from build123d import *
from OCP.BRepFilletAPI import BRepFilletAPI_MakeChamfer

# Parameters (mm, degrees)
BOSS_EXTRUDE1_DEPTH         = 2.29
SKETCH3_W                   = 0.64
SKETCH3_H                   = 0.64
CHAMFER3_SIZE               = 0.5
CHAMFER3_SIZE2              = 0.133974596
LPATTERN1_COUNT             = 5
LPATTERN1_PITCH             = 2.54
CHAMFER3_OF_LPATTERN1_SIZE  = 0.5
CHAMFER3_OF_LPATTERN1_SIZE2 = 0.133974596


with BuildPart() as part:
    # Sketch1 → Boss-Extrude1 (new body)
    with BuildSketch(Plane(origin=(0, 0, 0), x_dir=(1, 0, 0), z_dir=(0, 1, 0))):
        Polygon((-0.77, 1.25), (0.77, 1.25), (1.25, 0.75), (1.27, 0.75), (1.27, -0.75), (1.25, -0.75), (0.77, -1.25), (-0.77, -1.25), (-1.25, -0.75), (-1.27, -0.75), (-1.27, 0.75), (-1.25, 0.75), align=None)
    boss_extrude1 = extrude(amount=BOSS_EXTRUDE1_DEPTH)

    # Sweep1: sweep along a path in Sketch2
    with BuildLine(Plane(origin=(0, 0, 0), x_dir=(0, 0, -1), z_dir=(1, 0, 0))) as sweep1_path:
        Line((0, 8.13), (0, -0.408142235))
        ThreePointArc((0, -0.408142235), (-0.095150584, -0.886496526), (-0.366116524, -1.292025712))
        Line((-0.366116524, -1.292025712), (-2.124090812, -3.05))
    # Sketch3 → Sweep1 (sweep)
    with BuildSketch(Plane(origin=(0, 8.13, 0), x_dir=(1, 0, 0), z_dir=(0, 1, 0))):
        Rectangle(SKETCH3_W, SKETCH3_H)
    sweep1 = sweep(path=sweep1_path.line)

    # Chamfer3: one chamfer whose edges measure the first distance from different faces: ONE call of the kernel's chamfer builder (chamfer() names one face for all edges)
    chamfer3_edges_1 = [part.edges().sort_by_distance(p)[0] for p in [
        (0.32, 8.13, 0),
    ]]
    chamfer3_side_1 = [part.faces().sort_by_distance(p)[0] for p in [
        (0.32, 5.21, 0),
    ]]
    chamfer3_edges_2 = [part.edges().sort_by_distance(p)[0] for p in [
        (0, 8.13, -0.32),
    ]]
    chamfer3_side_2 = [part.faces().sort_by_distance(p)[0] for p in [
        (0, 5.21, -0.32),
    ]]
    chamfer3_edges_3 = [part.edges().sort_by_distance(p)[0] for p in [
        (-0.32, 8.13, 0),
    ]]
    chamfer3_side_3 = [part.faces().sort_by_distance(p)[0] for p in [
        (-0.32, 5.21, 0),
    ]]
    chamfer3_edges_4 = [part.edges().sort_by_distance(p)[0] for p in [
        (0, 8.13, 0.32),
    ]]
    chamfer3_side_4 = [part.faces().sort_by_distance(p)[0] for p in [
        (0, 5.21, 0.32),
    ]]
    chamfer3 = BRepFilletAPI_MakeChamfer(part.part.solid().wrapped)
    for e in chamfer3_edges_1:
        chamfer3.Add(CHAMFER3_SIZE, CHAMFER3_SIZE2, e.wrapped, chamfer3_side_1[0].wrapped)  # the first distance lies on this face
    for e in chamfer3_edges_2:
        chamfer3.Add(CHAMFER3_SIZE, CHAMFER3_SIZE2, e.wrapped, chamfer3_side_2[0].wrapped)  # the first distance lies on this face
    for e in chamfer3_edges_3:
        chamfer3.Add(CHAMFER3_SIZE, CHAMFER3_SIZE2, e.wrapped, chamfer3_side_3[0].wrapped)  # the first distance lies on this face
    for e in chamfer3_edges_4:
        chamfer3.Add(CHAMFER3_SIZE, CHAMFER3_SIZE2, e.wrapped, chamfer3_side_4[0].wrapped)  # the first distance lies on this face
    add(Compound.cast(chamfer3.Shape()), mode=Mode.REPLACE)

    # LPattern1: Boss-Extrude1, Sweep1 ×5
    with Locations(*[(i * LPATTERN1_PITCH, 0, 0) for i in range(1, LPATTERN1_COUNT)]):
        add(boss_extrude1)
        add(sweep1)

    # Chamfer3 of LPattern1: one chamfer whose edges measure the first distance from different faces: ONE call of the kernel's chamfer builder (chamfer() names one face for all edges)
    chamfer3_of_lpattern1_edges_1 = [part.edges().sort_by_distance(p)[0] for p in [
        (2.86, 8.13, 0),
    ]]
    chamfer3_of_lpattern1_side_1 = [part.faces().sort_by_distance(p)[0] for p in [
        (2.86, 5.21, 0),
    ]]
    chamfer3_of_lpattern1_edges_2 = [part.edges().sort_by_distance(p)[0] for p in [
        (2.54, 8.13, -0.32),
    ]]
    chamfer3_of_lpattern1_side_2 = [part.faces().sort_by_distance(p)[0] for p in [
        (2.54, 5.21, -0.32),
    ]]
    chamfer3_of_lpattern1_edges_3 = [part.edges().sort_by_distance(p)[0] for p in [
        (2.22, 8.13, 0),
    ]]
    chamfer3_of_lpattern1_side_3 = [part.faces().sort_by_distance(p)[0] for p in [
        (2.22, 5.21, 0),
    ]]
    chamfer3_of_lpattern1_edges_4 = [part.edges().sort_by_distance(p)[0] for p in [
        (2.54, 8.13, 0.32),
    ]]
    chamfer3_of_lpattern1_side_4 = [part.faces().sort_by_distance(p)[0] for p in [
        (2.54, 5.21, 0.32),
    ]]
    chamfer3_of_lpattern1_edges_5 = [part.edges().sort_by_distance(p)[0] for p in [
        (5.4, 8.13, 0),
    ]]
    chamfer3_of_lpattern1_side_5 = [part.faces().sort_by_distance(p)[0] for p in [
        (5.4, 5.21, 0),
    ]]
    chamfer3_of_lpattern1_edges_6 = [part.edges().sort_by_distance(p)[0] for p in [
        (5.08, 8.13, -0.32),
    ]]
    chamfer3_of_lpattern1_side_6 = [part.faces().sort_by_distance(p)[0] for p in [
        (5.08, 5.21, -0.32),
    ]]
    chamfer3_of_lpattern1_edges_7 = [part.edges().sort_by_distance(p)[0] for p in [
        (4.76, 8.13, 0),
    ]]
    chamfer3_of_lpattern1_side_7 = [part.faces().sort_by_distance(p)[0] for p in [
        (4.76, 5.21, 0),
    ]]
    chamfer3_of_lpattern1_edges_8 = [part.edges().sort_by_distance(p)[0] for p in [
        (5.08, 8.13, 0.32),
    ]]
    chamfer3_of_lpattern1_side_8 = [part.faces().sort_by_distance(p)[0] for p in [
        (5.08, 5.21, 0.32),
    ]]
    chamfer3_of_lpattern1_edges_9 = [part.edges().sort_by_distance(p)[0] for p in [
        (7.94, 8.13, 0),
    ]]
    chamfer3_of_lpattern1_side_9 = [part.faces().sort_by_distance(p)[0] for p in [
        (7.94, 5.21, 0),
    ]]
    chamfer3_of_lpattern1_edges_10 = [part.edges().sort_by_distance(p)[0] for p in [
        (7.62, 8.13, -0.32),
    ]]
    chamfer3_of_lpattern1_side_10 = [part.faces().sort_by_distance(p)[0] for p in [
        (7.62, 5.21, -0.32),
    ]]
    chamfer3_of_lpattern1_edges_11 = [part.edges().sort_by_distance(p)[0] for p in [
        (7.3, 8.13, 0),
    ]]
    chamfer3_of_lpattern1_side_11 = [part.faces().sort_by_distance(p)[0] for p in [
        (7.3, 5.21, 0),
    ]]
    chamfer3_of_lpattern1_edges_12 = [part.edges().sort_by_distance(p)[0] for p in [
        (7.62, 8.13, 0.32),
    ]]
    chamfer3_of_lpattern1_side_12 = [part.faces().sort_by_distance(p)[0] for p in [
        (7.62, 5.21, 0.32),
    ]]
    chamfer3_of_lpattern1_edges_13 = [part.edges().sort_by_distance(p)[0] for p in [
        (10.48, 8.13, 0),
    ]]
    chamfer3_of_lpattern1_side_13 = [part.faces().sort_by_distance(p)[0] for p in [
        (10.48, 5.21, 0),
    ]]
    chamfer3_of_lpattern1_edges_14 = [part.edges().sort_by_distance(p)[0] for p in [
        (10.16, 8.13, -0.32),
    ]]
    chamfer3_of_lpattern1_side_14 = [part.faces().sort_by_distance(p)[0] for p in [
        (10.16, 5.21, -0.32),
    ]]
    chamfer3_of_lpattern1_edges_15 = [part.edges().sort_by_distance(p)[0] for p in [
        (9.84, 8.13, 0),
    ]]
    chamfer3_of_lpattern1_side_15 = [part.faces().sort_by_distance(p)[0] for p in [
        (9.84, 5.21, 0),
    ]]
    chamfer3_of_lpattern1_edges_16 = [part.edges().sort_by_distance(p)[0] for p in [
        (10.16, 8.13, 0.32),
    ]]
    chamfer3_of_lpattern1_side_16 = [part.faces().sort_by_distance(p)[0] for p in [
        (10.16, 5.21, 0.32),
    ]]
    chamfer3_of_lpattern1 = BRepFilletAPI_MakeChamfer(part.part.solid().wrapped)
    for e in chamfer3_of_lpattern1_edges_1:
        chamfer3_of_lpattern1.Add(CHAMFER3_OF_LPATTERN1_SIZE, CHAMFER3_OF_LPATTERN1_SIZE2, e.wrapped, chamfer3_of_lpattern1_side_1[0].wrapped)  # the first distance lies on this face
    for e in chamfer3_of_lpattern1_edges_2:
        chamfer3_of_lpattern1.Add(CHAMFER3_OF_LPATTERN1_SIZE, CHAMFER3_OF_LPATTERN1_SIZE2, e.wrapped, chamfer3_of_lpattern1_side_2[0].wrapped)  # the first distance lies on this face
    for e in chamfer3_of_lpattern1_edges_3:
        chamfer3_of_lpattern1.Add(CHAMFER3_OF_LPATTERN1_SIZE, CHAMFER3_OF_LPATTERN1_SIZE2, e.wrapped, chamfer3_of_lpattern1_side_3[0].wrapped)  # the first distance lies on this face
    for e in chamfer3_of_lpattern1_edges_4:
        chamfer3_of_lpattern1.Add(CHAMFER3_OF_LPATTERN1_SIZE, CHAMFER3_OF_LPATTERN1_SIZE2, e.wrapped, chamfer3_of_lpattern1_side_4[0].wrapped)  # the first distance lies on this face
    for e in chamfer3_of_lpattern1_edges_5:
        chamfer3_of_lpattern1.Add(CHAMFER3_OF_LPATTERN1_SIZE, CHAMFER3_OF_LPATTERN1_SIZE2, e.wrapped, chamfer3_of_lpattern1_side_5[0].wrapped)  # the first distance lies on this face
    for e in chamfer3_of_lpattern1_edges_6:
        chamfer3_of_lpattern1.Add(CHAMFER3_OF_LPATTERN1_SIZE, CHAMFER3_OF_LPATTERN1_SIZE2, e.wrapped, chamfer3_of_lpattern1_side_6[0].wrapped)  # the first distance lies on this face
    for e in chamfer3_of_lpattern1_edges_7:
        chamfer3_of_lpattern1.Add(CHAMFER3_OF_LPATTERN1_SIZE, CHAMFER3_OF_LPATTERN1_SIZE2, e.wrapped, chamfer3_of_lpattern1_side_7[0].wrapped)  # the first distance lies on this face
    for e in chamfer3_of_lpattern1_edges_8:
        chamfer3_of_lpattern1.Add(CHAMFER3_OF_LPATTERN1_SIZE, CHAMFER3_OF_LPATTERN1_SIZE2, e.wrapped, chamfer3_of_lpattern1_side_8[0].wrapped)  # the first distance lies on this face
    for e in chamfer3_of_lpattern1_edges_9:
        chamfer3_of_lpattern1.Add(CHAMFER3_OF_LPATTERN1_SIZE, CHAMFER3_OF_LPATTERN1_SIZE2, e.wrapped, chamfer3_of_lpattern1_side_9[0].wrapped)  # the first distance lies on this face
    for e in chamfer3_of_lpattern1_edges_10:
        chamfer3_of_lpattern1.Add(CHAMFER3_OF_LPATTERN1_SIZE, CHAMFER3_OF_LPATTERN1_SIZE2, e.wrapped, chamfer3_of_lpattern1_side_10[0].wrapped)  # the first distance lies on this face
    for e in chamfer3_of_lpattern1_edges_11:
        chamfer3_of_lpattern1.Add(CHAMFER3_OF_LPATTERN1_SIZE, CHAMFER3_OF_LPATTERN1_SIZE2, e.wrapped, chamfer3_of_lpattern1_side_11[0].wrapped)  # the first distance lies on this face
    for e in chamfer3_of_lpattern1_edges_12:
        chamfer3_of_lpattern1.Add(CHAMFER3_OF_LPATTERN1_SIZE, CHAMFER3_OF_LPATTERN1_SIZE2, e.wrapped, chamfer3_of_lpattern1_side_12[0].wrapped)  # the first distance lies on this face
    for e in chamfer3_of_lpattern1_edges_13:
        chamfer3_of_lpattern1.Add(CHAMFER3_OF_LPATTERN1_SIZE, CHAMFER3_OF_LPATTERN1_SIZE2, e.wrapped, chamfer3_of_lpattern1_side_13[0].wrapped)  # the first distance lies on this face
    for e in chamfer3_of_lpattern1_edges_14:
        chamfer3_of_lpattern1.Add(CHAMFER3_OF_LPATTERN1_SIZE, CHAMFER3_OF_LPATTERN1_SIZE2, e.wrapped, chamfer3_of_lpattern1_side_14[0].wrapped)  # the first distance lies on this face
    for e in chamfer3_of_lpattern1_edges_15:
        chamfer3_of_lpattern1.Add(CHAMFER3_OF_LPATTERN1_SIZE, CHAMFER3_OF_LPATTERN1_SIZE2, e.wrapped, chamfer3_of_lpattern1_side_15[0].wrapped)  # the first distance lies on this face
    for e in chamfer3_of_lpattern1_edges_16:
        chamfer3_of_lpattern1.Add(CHAMFER3_OF_LPATTERN1_SIZE, CHAMFER3_OF_LPATTERN1_SIZE2, e.wrapped, chamfer3_of_lpattern1_side_16[0].wrapped)  # the first distance lies on this face
    add(Compound.cast(chamfer3_of_lpattern1.Shape()), mode=Mode.REPLACE)


solid = part.part
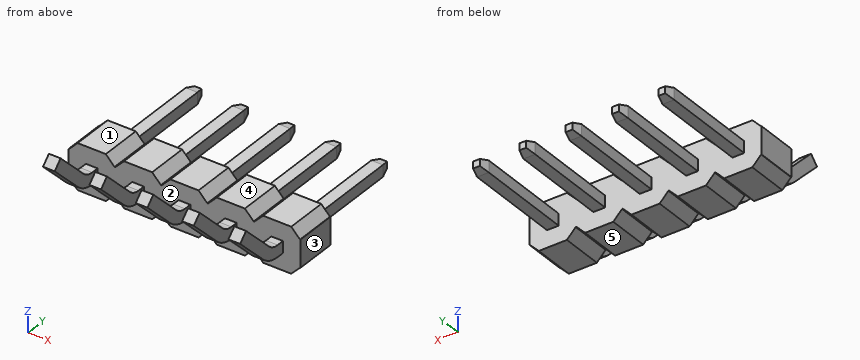
Design review of the part built by this model. Coordinates are the model's own, in mm. Face numbers are marked on the shaded views. A direction names the side the tool comes from. Give positions to 0.01 mm unless a question says otherwise; leave off trailing zeros. Loops run counter-clockwise (first coordinate to the right, second up) from the corner with the lowest first, then second, coordinate; pieces in that order, holes last. Notation, with made-up numbers: (13, 81.25) - (45, 81.25) arc R35 cw to (45, 115.25) - close; hole circle Ø8 at (-38.5, 19). An arc over 180 degrees is marked (long way). Use CSV: the item, a comma, the result in double quotes. Start each with the question number.
1. Add section B-B (x = 4.5). State the section outline as (y, z) points, plus the area to 4 significant figures.
2. Wall thickness on L1, parallel to X at y = 3, z = 0.1; L2, parallel to Y at x = 2, z = 0.8; L3, parallel to Z at x = 7.25, y = 1.75: over which ranges is each line inside the solid? List them lowest first.
3. Machinability: for the marked faces 4 and 5, which of the approach directions +Z, -Z, +X, -X, +Y, -Y give a long, thin tool a straight path to every point of the face, cutting with its end or side? Answer none if there is none.
4. Add section D-D (z = -0.6). State the section outline as (x, y) points, plus the area to 3 significant figures.
5. Add section C-C (y = -2.5). State the section outline as (x, z) points.
6. Draft analysis for pull direction X (two halves, no side actions). For the marked faces 1, 2 and 3, state which applies: released by +X, released by -X, zero draft, split by the parting line, or undercut.
7. Add section A-A (y = 2.5). State the section outline as (x, z) points, plus the area to 3 significant figures.
8. Insertion check: P1, Ø0.5, axis at x = 10.5, y = 5, coming from the +Z side; P2, Ø2, axis at x = 4.5, z = 1.5, coming from the +Y side; P3, Ø0.5, axis at y = 5, z = 0, coming from the +X side. Each pin has a flat end and moves straight along its axis. Give the tip position at first contact, or say it passes through.
Results found:
1,outline,"(0, -1.25) - (2.29, -1.25) - (2.29, 1.25) - (0, 1.25) - close"
1,area,"5.725 mm²"
2,L1,"x = -0.32 to 0.32, 2.22 to 2.86, 4.76 to 5.4, 7.3 to 7.94, 9.84 to 10.48"
2,L2,"y = 0 to 2.29"
2,L3,"z = -1.25 to 1.25"
3,face 4,"+Z, +X, -X, +Y"
3,face 5,"-Z, +X, -X, +Y, -Y"
4,outline,"(-1.27, 0) - (11.43, 0) - (11.43, 2.29) - (-1.27, 2.29) - close"
4,area,"29.1 mm²"
5,outline,"(-0.32, 1.12) - (0.32, 1.12) - (0.32, 2.03) - (-0.32, 2.03) - close; (2.22, 1.12) - (2.86, 1.12) - (2.86, 2.03) - (2.22, 2.03) - close; (4.76, 1.12) - (5.4, 1.12) - (5.4, 2.03) - (4.76, 2.03) - close; (7.3, 1.12) - (7.94, 1.12) - (7.94, 2.03) - (7.3, 2.03) - close; (9.84, 1.12) - (10.48, 1.12) - (10.48, 2.03) - (9.84, 2.03) - close"
6,face 1,"zero draft"
6,face 2,"undercut"
6,face 3,"released by +X"
7,outline,"(-0.32, -0.32) - (0.32, -0.32) - (0.32, 0.32) - (-0.32, 0.32) - close; (2.22, -0.32) - (2.86, -0.32) - (2.86, 0.32) - (2.22, 0.32) - close; (4.76, -0.32) - (5.4, -0.32) - (5.4, 0.32) - (4.76, 0.32) - close; (7.3, -0.32) - (7.94, -0.32) - (7.94, 0.32) - (7.3, 0.32) - close; (9.84, -0.32) - (10.48, -0.32) - (10.48, 0.32) - (9.84, 0.32) - close"
7,area,"2.05 mm²"
8,P1,"stops at z = 0.32"
8,P2,"stops at y = 2.29"
8,P3,"stops at x = 10.48"
